Design review of the part shown in the three views and the two pictorial views. Dimensions are in mm from the part's minimum x, y and z. A direction names the side the tool comes from. Coordinates: 2 decimals unless noted, no trailing zeros. Loops run counter-clockwise (first coordinate to the right, second up) from the corner with the lowest first, then second, coordinate; pieces in that order, holes last. Notation, with made-up numbers: (-26, 27) -> (-21, 27) arc R22 ccw to (-21, 42) -> close; hole circle Ø6 at (-0.75, 1.5). An arc over 180 degrees is marked (long way). One line per item, written item: value.
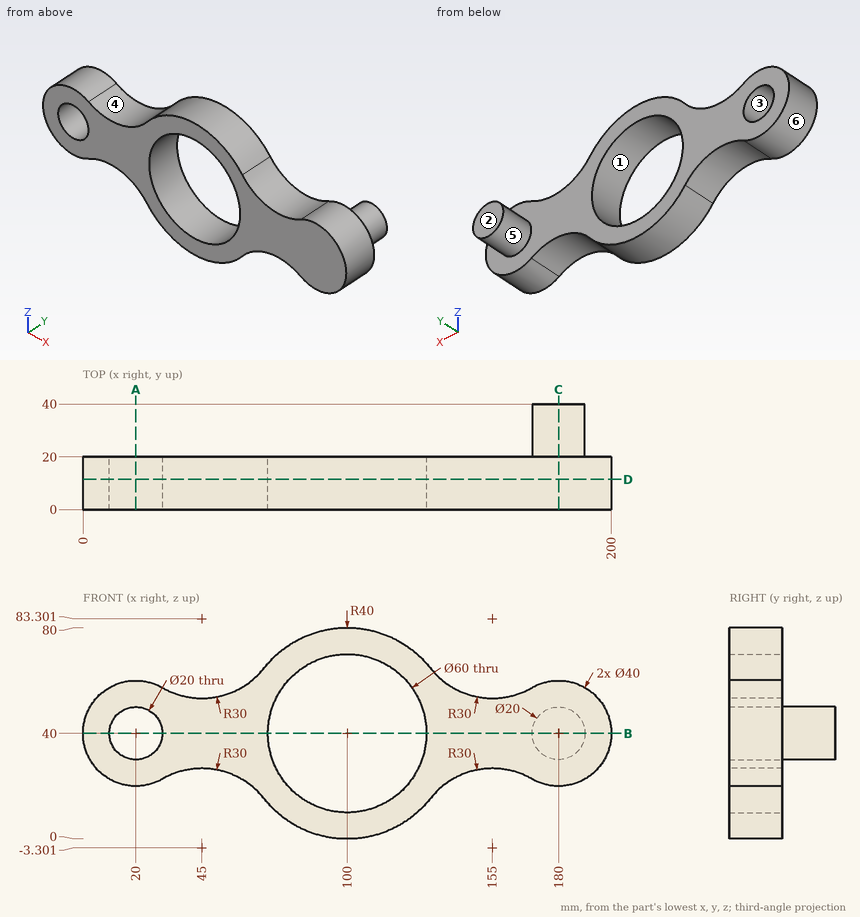
1. Insertion check: pin 1 Ø2 at (y, z) = (10, 49.5) entering from +X; pin 2 Ø10 at (y, z) = (34.5, 37) entering from -X; pin 3 Ø1.5 at (x, y) = (31.5, 14) entering from +Z. Each pin has a flat end and moves straight along its axis. Give the tip position at first contact, or say it passes through.
Return value:
pin 1: stops at x = 198.1
pin 2: stops at x = 170
pin 3: stops at z = 56.9
2. For the marked faces 5 and 6, list the 3-axis set-ups (+Z, -Z, +X, -X, +Y, -Y) from which the entire face can be reached by the end or side of a thin tool; tool diameter is ignored.
Return value:
face 5: +Y
face 6: +Y, -Y
3. Take a section at C-C, the plane x = 180. Give the boundary of the cut face in (y, z), and give its area (3 significant figures).
Return value:
outline: (0, 20) -> (20, 20) -> (20, 30) -> (40, 30) -> (40, 50) -> (20, 50) -> (20, 60) -> (0, 60) -> close
area: 1,200 mm2
4. Take a section at A-A, the plane x = 20. Give the boundary of the cut face in (y, z), and give its area (3 significant figures).
Return value:
outline: (0, 20) -> (20, 20) -> (20, 30) -> (0, 30) -> close; (0, 50) -> (20, 50) -> (20, 60) -> (0, 60) -> close
area: 400 mm2
5. The part is to be moulded in two halves that separate along Z. For the marked faces 1, 2, 3 and 4, say which applies: pulls with the +Z half, pulls with the -Z half, needs draft (parallel to the pull), parting line crosses it, or undercut.
Return value:
face 1: undercut
face 2: needs draft
face 3: undercut
face 4: pulls with the +Z half
6. Take a section at B-B, the plane z = 40. Give the boundary of the cut face in (x, y), and give its area (3 significant figures).
Return value:
outline: (0, 0) -> (10, 0) -> (10, 20) -> (0, 20) -> close; (30, 0) -> (70, 0) -> (70, 20) -> (30, 20) -> close; (130, 0) -> (200, 0) -> (200, 20) -> (190, 20) -> (190, 40) -> (170, 40) -> (170, 20) -> (130, 20) -> close
area: 2,800 mm2
7. Take a section at D-D, the plane y = 11.5. Give the boundary of the cut face in (x, z).
Return value:
outline: (30, 22.68) arc R30 cw to (68.57, 15.26) arc R40 ccw to (131.43, 15.26) arc R30 cw to (170, 22.68) arc R20 ccw (long way) to (170, 57.32) arc R30 cw to (131.43, 64.74) arc R40 ccw to (68.57, 64.74) arc R30 cw to (30, 57.32) arc R20 ccw (long way) to start; hole circle Ø20 at (20, 40); hole circle Ø60 at (100, 40)
8. To check wall thickness, follow probe 1 along Z at (x, y) = (20, 10.25); probe 2 along Y at (x, z) = (80.5, 64.5); probe 3 along Z at (x, y) = (100, 7). State the ranges of each line that lie inside material, in increasing order. Write a range as from..to.
Return value:
probe 1: z = 20..30, 50..60
probe 2: y = 0..20
probe 3: z = 0..10, 70..80
